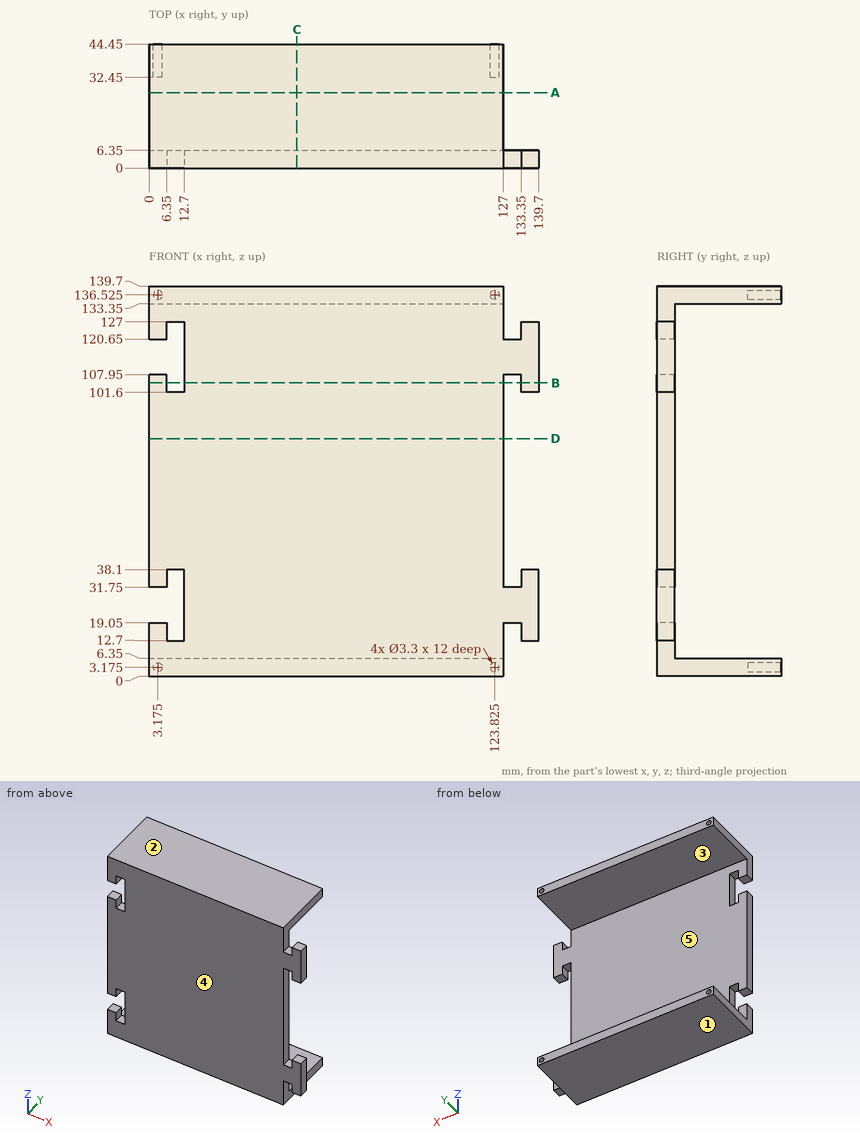
Source: three-view drawing plus pictorial views. Frame: mm from the lowest corner of the part. A direction names the side the tool comes from. Coordinates: 2 decimals unless noted, no trailing zeros. Write each loop counter-clockwise with the first axis right and the second up, starting at its lowest first coordinate (ties: lowest second). Pieces come first, ordered by that corner, then holes. Notation, with made-up numbers: (71.25, 47) -> (80.25, 47) arc R21 cw to (80.25, 62) -> close; hole circle Ø9 at (17.5, -16.75). An arc over 180 degrees is marked (long way). Answer as a JSON object with one key per item and string values.
1. Section A-A on y = 27. Return the cut outline in (x, z).
Result set:
{"outline": "(0, 0) -> (127, 0) -> (127, 6.35) -> (0, 6.35) -> close; (0, 133.35) -> (127, 133.35) -> (127, 139.7) -> (0, 139.7) -> close"}
2. Section D-D on z = 85. Return the cut outline in (x, y), then the cut area to 3 significant figures.
Result set:
{"outline": "(0, 0) -> (127, 0) -> (127, 6.35) -> (0, 6.35) -> close", "area": "806 mm2"}
3. Section C-C on x = 53. Return the cut outline in (y, z), then the cut area to 3 significant figures.
Result set:
{"outline": "(0, 0) -> (44.45, 0) -> (44.45, 6.35) -> (6.35, 6.35) -> (6.35, 133.35) -> (44.45, 133.35) -> (44.45, 139.7) -> (0, 139.7) -> close", "area": "1,370 mm2"}
4. Section B-B on z = 105. Return the cut outline in (x, y), then the cut area to 3 significant figures.
Result set:
{"outline": "(0, 0) -> (6.35, 0) -> (6.35, 6.35) -> (0, 6.35) -> close; (12.7, 0) -> (127, 0) -> (127, 6.35) -> (12.7, 6.35) -> close; (133.35, 0) -> (139.7, 0) -> (139.7, 6.35) -> (133.35, 6.35) -> close", "area": "806 mm2"}
5. First-contact query: P1, Ø1.7, axis at x = 123.5, z = 136.5, coming from the +Y side; P2, Ø3, axis at y = 3.5, z = 21.5, coming from the -X side; P3, Ø3, axis at x = 129.5, y = 4, coming from the -Z side. Flat tips, straight axial feed; report the tip coordinate or a pass-through.
Result set:
{"P1": "stops at y = 32.45", "P2": "stops at x = 12.7", "P3": "stops at z = 19.05"}
6. Material intervals for line 1 (Z direction, x = 50.5, y = 41); line 2 (Y direction, x = 80, z = 11.5), sorted ascending. Write a range as from..to.
Result set:
{"line 1": "z = 0..6.35, 133.35..139.7", "line 2": "y = 0..6.35"}
7. Access query for the marked faces 4 and 5. Directions: +Z, -Z, +X, -X, +Y, -Y. A direction counts if a zero-diameter tool reaches every point of the face in a straight line with its end or side. Return the directions, or none.
Result set:
{"face 4": "+Z, -Z, +X, -X, -Y", "face 5": "+X, -X, +Y"}
8. Mould query, pull axis Z, two halves, no side actions, for the marked faces 1, 2 and 3. Classes: released by +Z, released by -Z, zero draft, split by the parting line, or undercut.
Result set:
{"face 1": "released by -Z", "face 2": "released by +Z", "face 3": "undercut"}
